```python
from build123d import *

# Parameters (mm, degrees)
CYLINDER497_R          = 16.1
CYLINDER497_DEPTH      = 7
CYLINDER499_R          = 50
CYLINDER499_DEPTH      = 1.2
CYLINDER498_R          = 16.9
CYLINDER498_DEPTH      = 7
CUT238_PLACEMENT_ANGLE = 180


with BuildPart() as cylinder497:
    # Cylinder497 → Cylinder497 (new body)
    with BuildSketch(Plane.XY):
        Circle(CYLINDER497_R)
    extrude(amount=CYLINDER497_DEPTH)


with BuildPart() as cylinder499:
    # Cylinder499 → Cylinder499 (new body)
    with BuildSketch(Plane.XY):
        Circle(CYLINDER499_R)
    extrude(amount=CYLINDER499_DEPTH)


with BuildPart() as blades_top:
    # Cylinder498 → Cylinder498 (new body)
    with BuildSketch(Plane.XY):
        Circle(CYLINDER498_R)
    extrude(amount=CYLINDER498_DEPTH)

    # Fusion255: union Cylinder499
    add(cylinder499.part)

    # Cut238: cut Cylinder497
    add(cylinder497.part, mode=Mode.SUBTRACT)


with BuildPart() as blades_top_1:
    # Cut238 placement: moved
    add(blades_top.part.moved(Location((0, 0, 112.2))).rotate(Axis((0, 0, 112.2), (1, 0, 0)), CUT238_PLACEMENT_ANGLE))


solid = blades_top_1.part
```
Geometry check sheet. Reference: the model listing, model coordinates, mm. A direction names the side the tool comes from. Give positions to 0.01 mm unless a question says otherwise; leave off trailing zeros. Loops run counter-clockwise (first coordinate to the right, second up) from the corner with the lowest first, then second, coordinate; pieces in that order, holes last. Notation, with made-up numbers: (34, -15) - (50, -15) arc R16 cw to (50, -1) - close; hole circle Ø5 at (88.5, 2). An arc over 180 degrees is marked (long way). Use CSV: the item, a comma, the result in double quotes. Start each with the question number.
Q1. Scan lines: probe 1 along Y at (x, z) = (0, 108.5); probe 2 along Z at (x, y) = (-17, 22.5). Record each from-to range of solid material in increasing order. Write a range as from..to.
Q2. Section check C-C, the plane z = 107.75. Record the cut outline in (x, y), and give its area (3 significant figures).
Q3. Section check D-D, the plane x = 19.5. Record the cut outline in (y, z), and give its area (3 significant figures).
Q4. Go/stop test with flat-tipped pins: pin 1 Ø1.5 at (y, z) = (-6, 107) entering from -X; pin 2 Ø3 at (y, z) = (20, 108.5) entering from +X. Record where each tip stops, or that it passes through.
Q5. Release check for a two-part mould opening along Y. For faces 1 (the face through (47.69, -15.02, 111.61)), 2 (the face through (15.357, -4.836, 108.749)), 3 (the face through (-12, -12, 112.2)) record: +Y half, -Y half, draft (parallel to the pull), parting line (faces both ways), or undercut.
Q6. Section check A-A, the plane y = 0. Record the cut outline in (x, z).
Q7. Access from +Z, -Z, +X, -X, +Y, -Y to the whole of each face (thin tool, end or side, straight path). Record for faces 4 (the face through (16.12, -5.08, 108.14)), 5 (the face through (9, 14, 105.2)).
Findings below:
1,probe 1,"y = -16.9..-16.1, 16.1..16.9"
1,probe 2,"z = 111..112.2"
2,outline,"circle Ø33.8 at (0, 0); hole circle Ø32.2 at (0, 0)"
2,area,"82.9 mm^2"
3,outline,"(-46.04, 111) - (46.04, 111) - (46.04, 112.2) - (-46.04, 112.2) - close"
3,area,"110 mm^2"
4,pin 1,"stops at x = -16.06"
4,pin 2,"passes through"
5,face 1,"parting line"
5,face 2,"undercut"
5,face 3,"draft"
6,outline,"(-50, 111) - (-16.9, 111) - (-16.9, 105.2) - (-16.1, 105.2) - (-16.1, 112.2) - (-50, 112.2) - close; (16.1, 105.2) - (16.9, 105.2) - (16.9, 111) - (50, 111) - (50, 112.2) - (16.1, 112.2) - close"
7,face 4,"-Z"
7,face 5,"-Z, +X, -X, +Y, -Y"
